Part print with two shaded views. Sizes in mm from the minimum x, y, z corner. A direction names the side the tool comes from. Give positions to 0.01 mm unless a question says otherwise; leave off trailing zeros. Order: outer loops, then holes, each group sorted by start corner. A loop starts at its lowest first (then second) coordinate and runs counter-clockwise, first axis right, second up. Notation, with made-up numbers: (-20, 61) -> (13, 61) arc R24 ccw to (13, 72) -> close; hole circle Ø9 at (-22.75, 9). An arc over 180 degrees is marked (long way). Write item = value, one per line. Start each with the question number.
Item 1: Band-saw the part on C-C on z = 11.5. Write the cut outline in (x, y), plus the area to 3 significant figures.
Item 2: Pull direction Y, two halves, no side cores. Call the marked faces 3, 4 and 5: +Y half, -Y half, draft (parallel to the pull), parting line (faces both ways), or undercut.
Item 3: Drill centre lines: line 1 along Y through (x, z) = (38, 6); line 2 along Y through (x, z) = (38, 22). Where is each one in solid material? Low to high.
Item 4: Band-saw the part on A-A on x = 38.1. Write the cut outline in (y, z).
Item 5: Flat gauge pins, fed straight in: P1, Ø5, axis at x = 42, z = 35.5, coming from the -Y side; P2, Ø8, axis at y = 19.5, z = 16.5, coming from the -X side; P3, Ø11.5, axis at x = 63.5, y = 38.1, coming from the +Z side; P4, Ø14.5, axis at x = 38.1, y = 63.5, coming from the +Z side. Where does each tip first touch, or does it go through?
Item 6: Tool access for the marked faces 1 and 2: list every direction of +Z, -Z, +X, -X, +Y, -Y with a clear straight run to the whole face (end or side of a thin tool).
Item 7: Band-saw the part on D-D on x = 12.7. Write the cut outline in (y, z).
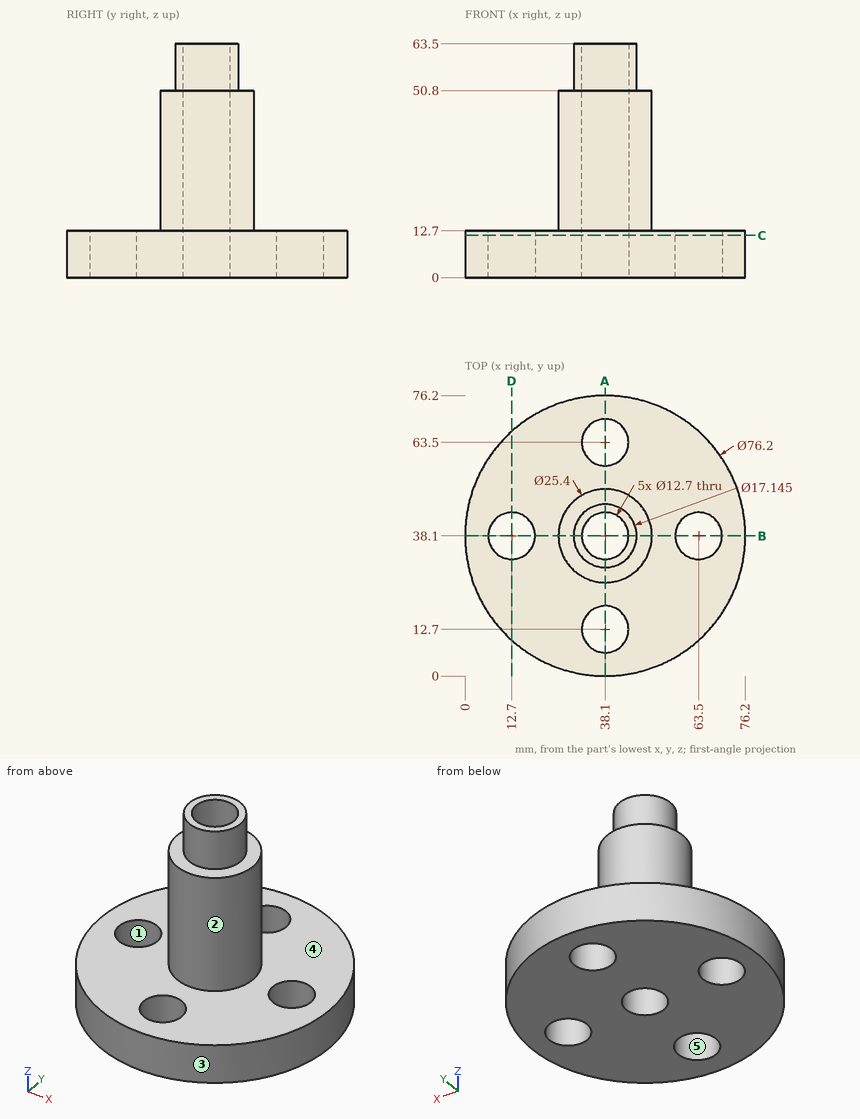
Values found:
q1.outline = circle Ø76.2 at (38.1, 38.1); hole circle Ø12.7 at (12.7, 38.1); hole circle Ø12.7 at (38.1, 12.7); hole circle Ø12.7 at (38.1, 38.1); hole circle Ø12.7 at (38.1, 63.5); hole circle Ø12.7 at (63.5, 38.1)
q1.area = 3,930 mm^2
q2.face_3 = parting line
q2.face_4 = draft
q2.face_5 = undercut
q3.line_1 = 0 to 6.35, 19.05 to 31.75, 44.45 to 57.15, 69.85 to 76.2
q3.line_2 = 25.4 to 31.75, 44.45 to 50.8
q4.outline = (0, 0) -> (6.35, 0) -> (6.35, 12.7) -> (0, 12.7) -> close; (19.05, 0) -> (31.75, 0) -> (31.75, 63.5) -> (29.53, 63.5) -> (29.53, 50.8) -> (25.4, 50.8) -> (25.4, 12.7) -> (19.05, 12.7) -> close; (44.45, 0) -> (57.15, 0) -> (57.15, 12.7) -> (50.8, 12.7) -> (50.8, 50.8) -> (46.67, 50.8) -> (46.67, 63.5) -> (44.45, 63.5) -> close; (69.85, 0) -> (76.2, 0) -> (76.2, 12.7) -> (69.85, 12.7) -> close
q5.P1 = 25.48
q5.P2 = 4.18
q5.P3 = through
q5.P4 = 12.7
q6.face_1 = +Z, -Z
q6.face_2 = +Z
q7.outline = (9.7, 0) -> (31.75, 0) -> (31.75, 12.7) -> (9.7, 12.7) -> close; (44.45, 0) -> (66.5, 0) -> (66.5, 12.7) -> (44.45, 12.7) -> close
